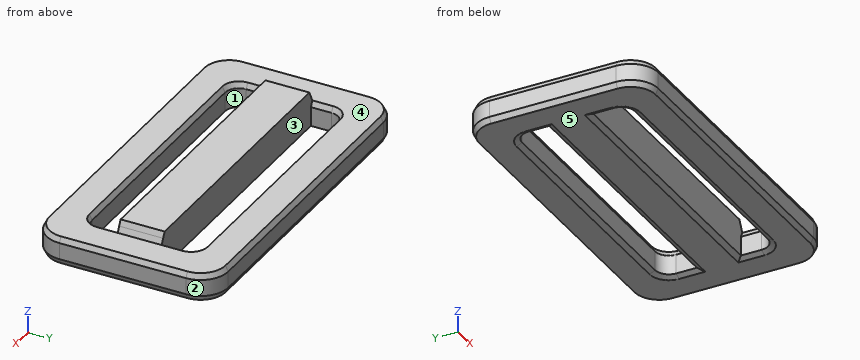
Autodesk Fusion 360 part; units mm, degrees
sketch "Sketch1" plane through (0, 0, 0) normal (0, 0, 1) x (1, 0, 0)
  line L0 (4, 0) -> (46, 0) construction
  line L1 (50, 0) -> (50, 22.4) construction
  line L2 (50, 26.4) -> (0, 26.4) construction
  line L3 (0, 22.4) -> (0, 0) construction
  line L4 (0, 13.2) -> (50, 13.2) construction
  line L5 (0, 16.4) -> (50, 16.4)
  line L6 (50, 16.4) -> (50, 13.2)
  line L7 (50, 13.2) -> (0, 13.2)
  line L8 (0, 13.2) -> (0, 16.4)
  line L9 (4, 26.4) -> (46, 26.4)
  line L10 (50, 26.4) -> (50, 4)
  line L11 (50, 0) -> (0, 0)
  line L12 (0, 4) -> (0, 26.4)
  line L13 (7, 5) -> (43, 5)
  line L14 (45, 7) -> (45, 19.4)
  line L15 (43, 21.4) -> (7, 21.4)
  line L16 (5, 19.4) -> (5, 7)
  line L17 (0, 10) -> (50, 10)
  arc A0 (4, 26.4) -> (0, 22.4) centre (4, 22.4) ccw
  arc A1 (0, 4) -> (4, 0) centre (4, 4) ccw
  arc A2 (46, 0) -> (50, 4) centre (46, 4) ccw
  arc A3 (50, 22.4) -> (46, 26.4) centre (46, 22.4) ccw
  arc A4 (7, 21.4) -> (5, 19.4) centre (7, 19.4) ccw
  arc A5 (5, 7) -> (7, 5) centre (7, 7) ccw
  arc A6 (43, 5) -> (45, 7) centre (43, 7) ccw
  arc A7 (45, 19.4) -> (43, 21.4) centre (43, 19.4) ccw
  line L18 (4.2, 16.4) -> (4.2, 10)
  line L19 (45.8, 16.4) -> (45.8, 10)
  point P0 (0, 13.2)
  dimension "d3" = 3.2
  dimension "d5" = 4
  dimension "d6" = 2
  dimension "d11" = 5
  dimension "d13" = 5
  dimension "d14" = 5
  dimension "d15" = 5
  dimension "d16" = 5
  dimension "d17" = 5
  dimension "d18" = 40
  dimension "d24" = 0.8
  dimension "d26" = 0.8
extrude "Extrude1" add sketch "Sketch1" along normal blind 4 contours L5 L9 L10 L12 L14 L15 L16 A0 A3 A4 A7 | L5 L7 L8 L12 L18 | L5 L7 L16 L18 | L7 L12 L17 L18 | L5 L7 L14 L16 | L7 L16 L17 L18 | L10 L11 L12 L13 L14 L16 L17 A1 A2 A5 A6 | L5 L7 L14 L19 | L7 L14 L16 L17 | L5 L6 L7 L10 L19 | L7 L14 L17 L19 | L7 L10 L17 L19
chamfer "Chamfer1" distance 0.4 distance2 0.8 38 edges at (44.4142, 20.8142, 0) (25, 21.4, 0) (5.5858, 20.8142, 0) (5, 17.9, 0) (45, 17.9, 0) (25, 5, 0) (44.4142, 5.5858, 0) (45, 8.5, 0) (5, 8.5, 0) (5.5858, 5.5858, 0) (25, 0, 0) (1.1716, 1.1716, 0) (0, 13.2, 0) (1.1716, 25.2284, 0) (25, 26.4, 0) (48.8284, 25.2284, 0) (50, 13.2, 0) (48.8284, 1.1716, 0) (25, 0, 4) (48.8284, 1.1716, 4) (50, 13.2, 4) (48.8284, 25.2284, 4) (25, 26.4, 4) (1.1716, 25.2284, 4) (0, 13.2, 4) (1.1716, 1.1716, 4) (25, 21.4, 4) (5.5858, 20.8142, 4) (5, 17.9, 4) (45, 17.9, 4) (44.4142, 20.8142, 4) (25, 5, 4) (44.4142, 5.5858, 4) (45, 8.5, 4) (5, 8.5, 4) (5.5858, 5.5858, 4) (25, 10, 0) (25, 16.4, 0) measured on face at (43.0952, 21.3977, 2.6667) measured on face at (31, 21.4, 1.3333) measured on face at (5.0023, 19.4952, 2.6667) measured on face at (5, 18.4, 1.3333) measured on face at (45, 17.4, 1.3333) measured on face at (19, 5, 1.3333) measured on face at (43.0952, 5.0023, 1.3333) measured on face at (45, 8, 1.3333) measured on face at (5, 9, 1.3333) measured on face at (5.1433, 6.2567, 2.6667) measured on face at (18.3333, 12.1333, 0) measured on face at (2.1671, 0.4447, 2.6667) measured on face at (18.3333, 12.1333, 0) measured on face at (0.22, 23.7083, 2.6667) measured on face at (18.3333, 12.1333, 0) measured on face at (49.4641, 24.4, 2.6667) measured on face at (18.3333, 12.1333, 0) measured on face at (46.943, 0.1128, 2.6667) measured on face at (18.3333, 12.1333, 4) measured on face at (18.3333, 12.1333, 4) measured on face at (18.3333, 12.1333, 4) measured on face at (18.3333, 12.1333, 4) measured on face at (18.3333, 12.1333, 4) measured on face at (18.3333, 12.1333, 4) measured on face at (18.3333, 12.1333, 4) measured on face at (18.3333, 12.1333, 4) measured on face at (18.3333, 12.1333, 4) measured on face at (18.3333, 12.1333, 4) measured on face at (18.3333, 12.1333, 4) measured on face at (18.3333, 12.1333, 4) measured on face at (18.3333, 12.1333, 4) measured on face at (18.3333, 12.1333, 4) measured on face at (18.3333, 12.1333, 4) measured on face at (18.3333, 12.1333, 4) measured on face at (18.3333, 12.1333, 4) measured on face at (18.3333, 12.1333, 4) measured on face at (18.3333, 10, 2.6667) measured on face at (18.3333, 16.4, 1.3333)
extrude "Extrude2" add sketch "Sketch1" along normal blind 1.6 from surface at 4 contours L5 L7 L14 L16 | L7 L14 L16 L17
chamfer "Chamfer2" distance 0.4 distance2 0.8 4 edges at (45, 13.2, 4) (5, 13.2, 4) (5, 13.2, 5.6) (45, 13.2, 5.6) measured on face at (19, 24.6, 4) measured on face at (19, 24.6, 4) measured on face at (18.3333, 14.2667, 5.6) measured on face at (18.3333, 14.2667, 5.6)
equation "d3 = ( 6.4 / 2 ) * 1 mm"
equation "d10 = Bevel_Horizontal"
equation "d11 = Linear Dimension-5"
equation "d13 = d11"
equation "d14 = d11"
equation "d15 = d11"
equation "d16 = d14"
equation "d17 = d14"
equation "d18 = Linear Dimension-9"
equation "d24 = Bevel_Horizontal"
equation "Bevel_Horizontal = 0.8 mm"
equation "d26 = Bevel_Horizontal"
equation "d28 = Bevel_Horizontal"
Design review of the part built by this model. Coordinates are the model's own, in mm. Face numbers are marked on the shaded views. A direction names the side the tool comes from. Coordinates: 2 decimals unless noted, no trailing zeros. Order: outer loops, then holes, each group sorted by start corner. A loop starts at its lowest first (then second) coordinate and runs counter-clockwise, first axis right, second up. Notation, with made-up numbers: (8, 31) -> (33, 31) arc R33 cw to (33, 68) -> close; hole circle Ø1 at (66, 37). An arc over 180 degrees is marked (long way). One line per item, written item: value. Start each with the question number.
Q1. Insertion check: pin 1 Ø1.5 at (x, z) = (20.5, 4) entering from +Y (3 decimals); pin 2 Ø6 at (x, y) = (8, 22) entering from +Z. Each pin has a flat end and moves straight along its axis. Give the tip position at first contact, or say it passes through.
Q2. For probe 1 along Y at (x, z) = (12.5, 1.7); probe 2 along X at (y, z) = (17, 2.1); probe 3 along Z at (x, y) = (47.5, 11.25), list the stretches that pass through material, from the lowest coordinate up.
Q3. Mouldability with a two-part tool opening along Z and no side actions: class the marked faces 3, 4 and 5 as pulls with the +Z half, pulls with the -Z half, needs draft (parallel to the pull), parting line crosses it, or undercut.
Q4. Tool access review of the marked faces 1 and 2: name each direction out of +Z, -Z, +X, -X, +Y, -Y from which nothing blocks a thin tool from reaching the whole face with its end or side.
Q5. Take a section at A-A, the plane x = 8.5. State the section outline as (y, z) points, then the cut area to 3 significant figures.
Values follow:
1. pin 1: stops at y = 26.375
1. pin 2: stops at z = 4
2. probe 1: y = 0 to 5, 10 to 16.4, 21.4 to 26.4
2. probe 2: x = 0 to 5, 45 to 50
2. probe 3: z = 0 to 4
3. face 3: needs draft
3. face 4: pulls with the +Z half
3. face 5: pulls with the -Z half
4. face 1: +Z, -Z
4. face 2: +Z, -Z, +X, +Y
5. outline: (0, 0.8) -> (0.4, 0) -> (4.2, 0) -> (5, 0.4) -> (5, 3.2) -> (4.6, 4) -> (0.4, 4) -> (0, 3.2) -> close; (10, 0.4) -> (10.8, 0) -> (15.6, 0) -> (16.4, 0.4) -> (16.4, 5.6) -> (10, 5.6) -> close; (21.4, 0.4) -> (22.2, 0) -> (26, 0) -> (26.4, 0.8) -> (26.4, 3.2) -> (26, 4) -> (21.8, 4) -> (21.4, 3.2) -> close
5. area: 74.2 mm2
